Build history of the part. All positions in model axes, mm. Round coordinates to 2 decimals unless told otherwise and drop trailing zeros. Order: outer loops, then holes, each group sorted by start corner. A loop starts at its lowest first (then second) coordinate and runs counter-clockwise, first axis right, second up. Notation, with made-up numbers: (54.25, -22.75) -> (63.25, -22.75) arc R28 ccw to (63.25, -2.75) -> close; hole circle Ø5 at (89.25, 61.25). An arc over 180 degrees is marked (long way). Write item = value, one per line.
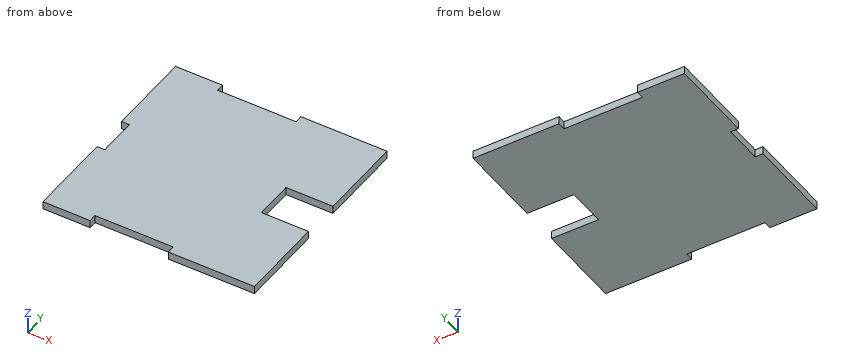
from build123d import *

# Parameters (mm, degrees)
SKETCH2_W           = 108
SKETCH2_H           = 108
BOSS_EXTRUDE1_DEPTH = 4
SKETCH3_W           = 20
SKETCH3_H           = 8
SKETCH3_W_2         = 8
SKETCH3_H_2         = 20
CUT_EXTRUDE1_DEPTH  = 4
SKETCH4_W           = 20
SKETCH4_H           = 4
SKETCH4_H_2         = 20
CUT_EXTRUDE2_DEPTH  = 4


with BuildPart() as part:
    # Sketch2 → Boss-Extrude1 (new body)
    with BuildSketch(Plane.XY):
        Rectangle(SKETCH2_W, SKETCH2_H)
    extrude(amount=BOSS_EXTRUDE1_DEPTH)

    # Sketch3 → Cut-Extrude1 (cut)
    with BuildSketch(Plane(origin=(0, 0, 0), x_dir=(-1, 0, 0), z_dir=(0, 0, -1))):
        with Locations((0, 54)):
            Rectangle(SKETCH3_W, SKETCH3_H)
        with Locations((54, 0)):
            Rectangle(SKETCH3_W_2, SKETCH3_H_2)
        with Locations((-54, 0)):
            Rectangle(SKETCH3_W_2, SKETCH3_H_2)
        with Locations((0, -54)):
            Rectangle(SKETCH3_W, SKETCH3_H)
    extrude(amount=-CUT_EXTRUDE1_DEPTH, mode=Mode.SUBTRACT)

    # Sketch4 → Cut-Extrude2 (cut)
    with BuildSketch(Plane(origin=(0, 0, 0), x_dir=(-1, 0, 0), z_dir=(0, 0, -1))):
        with Locations((20, 52)):
            Rectangle(SKETCH4_W, SKETCH4_H)
        with Locations((20, -52)):
            Rectangle(SKETCH4_W, SKETCH4_H)
        with Locations((-40, 0)):
            Rectangle(SKETCH4_W, SKETCH4_H_2)
    extrude(amount=-CUT_EXTRUDE2_DEPTH, mode=Mode.SUBTRACT)


solid = part.part
Q1. Probe probe 1 along Y at (x, z) = (33, 2.4); probe 2 along Y at (x, z) = (-26, 3). List the from-to ranges inside material, lowest first.
Check values:
probe_1 = -54 to -10, 10 to 54
probe_2 = -50 to 50
Q2. Cut at B-B, the plane x = -2. List the corners of the cut face in (y, z).
Check values:
outline = (-50, 0) -> (50, 0) -> (50, 4) -> (-50, 4) -> close
Q3. Cut at A-A, the plane z = 1.4. List the corners of the cut face in (x, y), and give its area (3 significant figures).
Check values:
outline = (-54, -54) -> (-30, -54) -> (-30, -50) -> (10, -50) -> (10, -54) -> (54, -54) -> (54, -10) -> (30, -10) -> (30, 10) -> (54, 10) -> (54, 54) -> (10, 54) -> (10, 50) -> (-30, 50) -> (-30, 54) -> (-54, 54) -> (-54, 10) -> (-50, 10) -> (-50, -10) -> (-54, -10) -> close
area = 10,800 mm²
Q4. Flat gauge pin, fed straight in: pin 1 (1.2 mm diameter, centred on x = -0.5, z = 2.5, fed in from +Y). Where does the tip first touch, or does it go through?
Check values:
pin_1 = 50
